Autodesk Inventor part; units mm, degrees
ref_plane "YZ Plane" through (0, 0, 0) normal (1, 0, 0) x (0, 1, 0)
ref_plane "XZ Plane" through (0, 0, 0) normal (0, 1, 0) x (-1, 0, 0)
ref_plane "XY Plane" through (0, 0, 0) normal (0, 0, 1) x (1, 0, 0)
sketch "Sketch1" plane through (0, 0, 0) normal (0, 0, 1) x (1, 0, 0)
  line L0 (0, 0) -> (27.94, 0)
  line L1 (27.94, 0) -> (27.94, 203.2)
  line L2 (0, 0) -> (-27.94, 0)
  line L3 (-27.94, 0) -> (-27.94, 203.2)
  line L4 (-27.94, 203.2) -> (-37.465, 203.2)
  line L5 (-37.465, 203.2) -> (-37.465, -9.525)
  line L6 (-37.465, -9.525) -> (37.465, -9.525)
  line L7 (37.465, -9.525) -> (37.465, 203.2)
  line L8 (37.465, 203.2) -> (27.94, 203.2)
  dimension "d0" = 203.2
  dimension "d1" = 27.94
  dimension "x2" = 9.525
  dimension "d3" = 9.525
  dimension "d4" = 9.525
extrude "Extrusion1" add sketch "Sketch1" against normal mid plane 76.2
sketch "Sketch2" plane through (37.465, -9.525, -38.1) normal (1, 0, 0) x (0, 0, -1)
  circle A0 centre (-38.1, 200.025) radius 7.9375
  point P0 (-38.1, 9.525)
  dimension "d7" = 15.875
  dimension "d8" = 190.5
extrude "Extrusion2" cut sketch "Sketch2" against normal through all
sketch "Sketch3" plane through (0, 0, 38.1) normal (0, 0, 1) x (1, 0, 0)
  line L0 (37.465, 203.2) -> (37.465, -9.525)
  line L1 (37.465, 132.461) -> (69.215, 132.461)
  line L2 (69.215, 132.461) -> (69.215, 113.411)
  line L3 (69.215, 113.411) -> (37.465, 113.411)
  line L4 (37.465, 113.411) -> (37.465, 132.461)
  line L5 (37.465, 122.936) -> (69.215, 122.936) construction
  line L6 (-37.465, -9.525) -> (37.465, -9.525) construction
  circle A0 centre (53.1368, 122.936) radius 4.7625
  point P0 (0, 0)
  point P1 (37.465, 113.411)
  dimension "d20" = 31.75
  dimension "d21" = 19.05
  dimension "d22" = 132.461
  dimension "d23" = 9.525
  dimension "d24" = 15.6718
extrude "Extrusion3" add sketch "Sketch3" against normal blind 19.05
mirror "Mirror1" about plane through (0, 0, 0) normal (0, 0, 1) of "Extrusion3"
sketch "Sketch4" plane through (-37.465, -9.525, -38.1) normal (0, -1, 0) x (1, 0, 0)
  circle A0 centre (37.465, 38.1) radius 20.6375
  dimension "d27" = 41.275
extrude "Extrusion4" cut sketch "Sketch4" against normal through all
equation "\"d0\" = overallHeight"
equation "\"x2\" = wallThickness"
equation "\"d3\" = wallThickness"
equation "\"d4\" = wallThickness"
equation "\"d5\" = overallWidth"
equation "\"d7\" = postHoleDiameter"
equation "\"postHoleDiameter\" = 15.875"
equation "\"overallHeight\" = 203.2"
equation "\"wallThickness\" = 9.525"
equation "\"overallWidth\" = 76.2"
properties part number "forkV02" material "PC/ABS Plastic"
Could you check a few things on this model? Use its own coordinates, in mm. A direction names the side the tool comes from. Give positions to 0.01 mm unless a question says otherwise; leave off trailing zeros. Write each loop counter-clockwise with the first axis right and the second up, starting at its lowest first coordinate (ties: lowest second). Pieces come first, ordered by that corner, then holes. Notation, with made-up numbers: (34, 38.5) -> (51, 38.5) arc R12 cw to (51, 48.5) -> close; hole circle Ø7 at (-16, 62.25). An arc over 180 degrees is marked (long way). Write each question's results on one line, items separated by ' | '.
1. If we mould it in two halves opening along Z, with no side actions, what happens to faces 1 (the flat face through (31, 82, 38.1)), 2 (the flat face through (-19, 0, 9)), 3 (the cylindrical face through (-4.474, -4.829, -20.147))? For each: released by +Z, released by -Z, zero draft, split by the parting line, or undercut.
Check sheet entries:
face 1: released by +Z | face 2: zero draft | face 3: undercut
2. I need wall thicknesses on L1, parallel to X at y = 2.5, z = -32 (3 decimals); L2, parallel to Y at x = -35, z = 0 (1 decimal); L3, parallel to Z at x = 0, y = -2. Which ranges of each line are inside material? Lowest first, please.
Check sheet entries:
L1: x = -37.465 to -27.94, 27.94 to 37.465 | L2: y = -9.5 to 182.6, 198.4 to 203.2 | L3: z = -38.1 to -20.64, 20.64 to 38.1
3. I want a section at D-D, the plane x = 0. Write out the boundary of the cut face in (y, z) (1 decimal).
Check sheet entries:
outline: (-9.5, -38.1) -> (0, -38.1) -> (0, -20.6) -> (-9.5, -20.6) -> close; (-9.5, 20.6) -> (0, 20.6) -> (0, 38.1) -> (-9.5, 38.1) -> close
4. I want a section at B-B, the plane z = 0. Write out the boundary of the cut face in (x, y) (1 decimal), then the cut area to 3 significant figures.
Check sheet entries:
outline: (-37.5, -9.5) -> (-20.6, -9.5) -> (-20.6, 0) -> (-27.9, 0) -> (-27.9, 182.6) -> (-37.5, 182.6) -> close; (-37.5, 198.4) -> (-27.9, 198.4) -> (-27.9, 203.2) -> (-37.5, 203.2) -> close; (20.6, -9.5) -> (37.5, -9.5) -> (37.5, 182.6) -> (27.9, 182.6) -> (27.9, 0) -> (20.6, 0) -> close; (27.9, 198.4) -> (37.5, 198.4) -> (37.5, 203.2) -> (27.9, 203.2) -> close | area: 3,890 mm²
5. Will these pins go through, and if not, where does the flat tip stop? pin 1 Ø8 at (x, z) = (47.5, 20.5) entering from +Y; pin 2 Ø5.5 at (x, y) = (53.14, 122.94) entering from +Z; pin 3 Ø9.5 at (x, z) = (50.5, 31) entering from -Y; pin 4 Ø18.5 at (y, z) = (190.5, 0) entering from +X (3 decimals).
Check sheet entries:
pin 1: stops at y = 132.46 | pin 2: passes through | pin 3: stops at y = 113.41 | pin 4: stops at x = 37.465
6. I want a section at C-C, the plane y = 38. Write out the boundary of the cut face in (x, z) (3 decimals).
Check sheet entries:
outline: (-37.465, -38.1) -> (-27.94, -38.1) -> (-27.94, 38.1) -> (-37.465, 38.1) -> close; (27.94, -38.1) -> (37.465, -38.1) -> (37.465, 38.1) -> (27.94, 38.1) -> close
7. I want a section at A-A, the plane y = 190.5. Write out the boundary of the cut face in (x, z) (1 decimal).
Check sheet entries:
outline: (-37.5, -38.1) -> (-27.9, -38.1) -> (-27.9, -7.9) -> (-37.5, -7.9) -> close; (-37.5, 7.9) -> (-27.9, 7.9) -> (-27.9, 38.1) -> (-37.5, 38.1) -> close; (27.9, -38.1) -> (37.5, -38.1) -> (37.5, -7.9) -> (27.9, -7.9) -> close; (27.9, 7.9) -> (37.5, 7.9) -> (37.5, 38.1) -> (27.9, 38.1) -> close
8. On a 3-axis mill with a long thin cutter (end or side, diameter ignored), from which of +Z, -Z, +X, -X, +Y, -Y can I reach the whole of each face in a straight line? I mean faces 4 (the flat face through (53, 113.411, -29)), 5 (the flat face through (-27.94, 100, 1)), 6 (the flat face through (50, 127, -19.05)), 7 (the flat face through (53, 132.461, 29)). Say none if no direction works.
Check sheet entries:
face 4: +Z, -Z, +X, -Y | face 5: +Z, -Z, +Y | face 6: +X, +Y, -Y | face 7: +Z, -Z, +X, +Y
